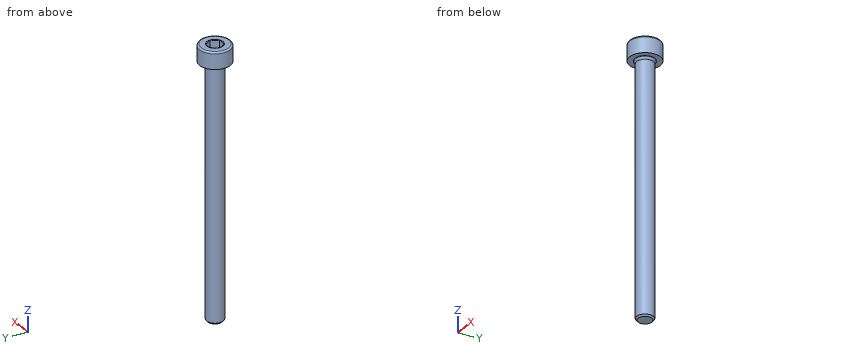
Solid Edge part; units mm, degrees
sketch "Sketch1" plane through (0, 0, 0) normal (0, 0, 1) x (1, 0, 0)
  line L0 (-0.7217, 1.25) -> (0.7217, 1.25)
  line L1 (0.7217, 1.25) -> (1.4434, 0)
  line L2 (1.4434, 0) -> (0.7217, -1.25)
  line L3 (0.7217, -1.25) -> (-0.7217, -1.25)
  line L4 (-0.7217, -1.25) -> (-1.4434, 0)
  line L5 (-1.4434, 0) -> (-0.7217, 1.25)
  circle A0 centre (0, 0) radius 2.75
extrude "Protrusion1" add sketch "Sketch1" along normal blind 3
sketch "Sketch2" plane through (0, 0, 0) normal (0, -1, 0) x (1, 0, 0)
  line L0 (0, 0.8667) -> (1.4434, 1.7)
  line L1 (1.4434, 1.7) -> (2.75, 1.7)
  line L2 (2.75, 1.7) -> (2.75, 0)
  line L3 (2.75, 0) -> (1.5, 0)
  line L4 (1.5, 0) -> (1.5, -26.999)
  line L5 (1.5, -26.999) -> (1.5, -27) construction
  line L6 (1.5, -27) -> (1.5, -27) construction
  line L7 (1.5, -27) -> (1.5, -45)
  line L8 (0, -45) -> (1.5, -45)
revolve "RevolvedProtrusion_1" add sketch "Sketch2" angle 360 about axis through (0, 0, 2.3333) along (0, 0, -1)
cosmetic_thread "Thread_1" thread depth 17.999
sketch "Sketch3" plane through (0, 0, 0) normal (0, -1, 0) x (1, 0, 0)
  line L0 (0, 4) -> (1.435, 4)
  line L1 (1.435, 4) -> (1.435, 3)
  line L2 (1.435, 3) -> (0, 2.1715)
revolve "RevolvedCutout_1" cut sketch "Sketch3" angle 360 about axis through (0, 0, 7.1999) along (0, 0, 1)
fillet "Round_1" radius 0.3 1 edges at (-2.75, 0, 3)
sketch "Sketch4" plane through (0, 0, 0) normal (0, -1, 0) x (1, 0, 0)
  line L0 (1.5, 0) -> (1.8, 0)
  arc A0 (1.7101, -0.0562) -> (1.8, 0) centre (1.8, -0.1) cw
  line L1 (1.5101, -0.4662) -> (1.7101, -0.0562)
  arc A1 (1.5101, -0.4662) -> (1.5, -0.51) centre (1.6, -0.51) ccw
  line L2 (1.5, 0) -> (1.5, -0.51)
revolve "RevolvedProtrusion_2" add sketch "Sketch4" angle 360 about axis through (0, 0, -1.02) along (0, 0, 1)
chamfer "Chamfer_1" distance 0.2705 angle 45 1 edges at (-1.5, 0, -45)
properties material "Steel"
Model file for the job. Use its own axes, mm. Coordinates: 2 decimals unless noted, no trailing zeros. Order: outer loops, then holes, each group sorted by start corner. A loop starts at its lowest first (then second) coordinate and runs counter-clockwise, first axis right, second up. Notation, with made-up numbers: (24.5, 36.25) - (36.5, 36.25) arc R15 ccw to (36.5, 65.25) - close; hole circle Ø6 at (-36, 38.5). An arc over 180 degrees is marked (long way). Return JSON: item names as keys, results as strings. Group by question number.
1) Probe line 1 (Y direction, x = -0.45, z = -25.5); line 2 (Z direction, x = 2.25, y = 0.1); line 3 (Z direction, x = 0.75, y = -1.35). List the from-to ranges inside material, lowest first. Write a range as from..to.
2) Saw through at A-A, the plane z = -5. Write the cut outline in (x, y), plus the area to 3 significant figures.
3) Flat gauge pins, fed straight in: P1, Ø3, axis at x = 0.5, z = -28, coming from the +Y side; P2, Ø3, axis at y = 1, z = -37.5, coming from the +X side. Where does each tip first touch, or does it go through?
Values found:
{
 "1": {"line 1": "y = -1.43..1.43", "line 2": "z = 0..3", "line 3": "z = -0.4..3"},
 "2": {"outline": "circle Ø3 at (0, 0)", "area": "7.07 mm²"},
 "3": {"P1": "stops at y = 1.5", "P2": "stops at x = 1.5"}
}
